```python
from build123d import *

# Parameters (mm, degrees)
SKETCH_1_R      = 1.3
EXTRUDE_1_DEPTH = 1.6
EXTRUDE_2_DEPTH = 6
SKETCH_3_W      = 6
SKETCH_3_H      = 6
EXTRUDE_3_DEPTH = 0.6
SKETCH_4_W      = 1.6
SKETCH_4_H      = 1.6
EXTRUDE_4_DEPTH = 0.6
SKETCH_5_W      = 32.8
SKETCH_5_H      = 9.5
EXTRUDE_5_DEPTH = 8


with BuildPart() as part:
    # 草图1 → 凸台-拉伸1 (new body)
    with BuildSketch(Plane(origin=(0, 0, 0), x_dir=(1, 0, 0), z_dir=(0, 1, 0))):
        with BuildLine():
            Line((-12, -17.5), (12, -17.5))
            ThreePointArc((12, -17.5), (12.707106781, -17.207106781), (13, -16.5))
            Line((13, -16.5), (13, 16.5))
            ThreePointArc((13, 16.5), (12.707106781, 17.207106781), (12, 17.5))
            Line((12, 17.5), (-12, 17.5))
            ThreePointArc((-12, 17.5), (-12.707106781, 17.207106781), (-13, 16.5))
            Line((-13, 16.5), (-13, -16.5))
            ThreePointArc((-13, -16.5), (-12.707106781, -17.207106781), (-12, -17.5))
        make_face()
        with Locations((-11, -15.5)):
            Circle(SKETCH_1_R, mode=Mode.SUBTRACT)
        with Locations((11, 15.5)):
            Circle(SKETCH_1_R, mode=Mode.SUBTRACT)
    extrude(amount=EXTRUDE_1_DEPTH)

    # 草图2 → 凸台-拉伸2 (add)
    with BuildSketch(Plane.ZY.offset(13)):
        with BuildLine():
            Line((-3.4, 3.2), (3.4, 3.2))
            ThreePointArc((3.4, 3.2), (5, 1.6), (3.4, 0))
            Line((3.4, 0), (-3.4, 0))
            ThreePointArc((-3.4, 0), (-5, 1.6), (-3.4, 3.2))
        make_face()
    extrude(amount=-EXTRUDE_2_DEPTH)

    # 草图3 → 凸台-拉伸3 (add)
    with BuildSketch(Plane(origin=(0, 1.6, 0), x_dir=(1, 0, 0), z_dir=(0, 1, 0))):
        with Locations((0.65, 0)):
            Rectangle(SKETCH_3_W, SKETCH_3_H)
    extrude(amount=EXTRUDE_3_DEPTH)

    # 草图4 → 凸台-拉伸4 (add)
    with BuildSketch(Plane(origin=(0, 1.6, 0), x_dir=(1, 0, 0), z_dir=(0, 1, 0))):
        with Locations((8.15, 0)):
            Rectangle(SKETCH_4_W, SKETCH_4_H)
    extrude(amount=EXTRUDE_4_DEPTH)

    # 草图5 → 凸台-拉伸5 (add)
    with BuildSketch(Plane(origin=(13, 0, 0), x_dir=(0, 0, -1), z_dir=(1, 0, 0))):
        with Locations((0, 0.8)):
            Rectangle(SKETCH_5_W, SKETCH_5_H)
    extrude(amount=EXTRUDE_5_DEPTH)


solid = part.part
```
CAD build for the part. Positions are in the model's coordinates, mm. A direction names the side the tool comes from. Round coordinates to 2 decimals unless told otherwise and drop trailing zeros. Write each loop counter-clockwise with the first axis right and the second up, starting at its lowest first coordinate (ties: lowest second). Pieces come first, ordered by that corner, then holes. Notation, with made-up numbers: (-32.75, -37.75) - (18.25, -37.75) arc R11 ccw to (18.25, -20.75) - close; hole circle Ø6 at (29, 64). An arc over 180 degrees is marked (long way). Write item = value, one per line. Start each with the question number.
Q1. Drop flat-ended pins along their axis: pin 1 (0.8 mm diameter, centred on x = 8, z = 0.5, fed in from +Y); pin 2 (4 mm diameter, centred on x = 16, y = 1.5, fed in from +Z); pin 3 (0.5 mm diameter, centred on x = -1, y = 2, fed in from +Z). Give the stop position or say it passes through.
Q2. Band-saw the part on B-B (x = -11). Give the cut face in (y, z), then the cut area to 3 significant figures.
Q3. Band-saw the part on D-D (x = 11). Give the cut face in (y, z).
Q4. Band-saw the part on A-A (z = -15.5). Give the cut face in (x, y).
Q5. Band-saw the part on C-C (z = -6). Give the cut face in (x, y), then the cut area to 3 significant figures.
Q6. Probe L1, parallel to X at y = 1.1, z = -15.5; L2, parallel to Z at x = 11, y = 1; L3, parallel to Z at x = -11, y = 1.05. List the from-to ranges inside material, lowest first. Write a range as from..to.
Q7. Mould opens along X. For faces 4 (the flat face through (13, 4, 0)), 5 (the flat face through (13, -2, 0)), 6 (the cylindrical face through (-10.04, 2.74, 4.52)), 7 (the flat face through (21, 1, 0)) say: pulls with the +X half, pulls with the -X half, needs draft (parallel to the pull), parting line crosses it, or undercut.
Q8. Which spindle directions (+Z, -Z, +X, -X, +Y, -Y) get a long thin tool onto all of the face, cutting with end or side? Do faces 1 (the cylindrical face through (-10.04, 2.72, -4.54)), 2 (the flat face through (-7, 2, 0)), 3 (the flat face through (17, -3.95, 0)). Say none if no direction does.
Answers below:
q1.pin_1 = 2.2
q1.pin_2 = 16.4
q1.pin_3 = 3
q2.outline = (0, -17.5) - (1.6, -17.5) - (1.6, -5) arc R1.6 ccw to (3.2, -3.4) - (3.2, 3.4) arc R1.6 ccw to (1.6, 5) - (1.6, 14.2) - (0, 14.2) - close; (0, 16.8) - (1.6, 16.8) - (1.6, 17.5) - (0, 17.5) - close
q2.area = 66.7 mm2
q3.outline = (0, -17.5) - (1.6, -17.5) - (1.6, -16.8) - (0, -16.8) - close; (0, -14.2) - (1.6, -14.2) - (1.6, 17.5) - (0, 17.5) - close
q4.outline = (-13, 0) - (9.7, 0) - (9.7, 1.6) - (-13, 1.6) - close; (12.3, 0) - (13, 0) - (13, -3.95) - (21, -3.95) - (21, 5.55) - (13, 5.55) - (13, 1.6) - (12.3, 1.6) - close
q5.outline = (-13, 0) - (13, 0) - (13, -3.95) - (21, -3.95) - (21, 5.55) - (13, 5.55) - (13, 1.6) - (-13, 1.6) - close
q5.area = 118 mm2
q6.L1 = -13..9.7, 12.3..21
q6.L2 = -17.5..-16.8, -14.2..17.5
q6.L3 = -17.5..14.2, 16.8..17.5
q7.face_4 = undercut
q7.face_5 = pulls with the -X half
q7.face_6 = needs draft
q7.face_7 = pulls with the +X half
q8.face_1 = -Z, -X, +Y
q8.face_2 = +Z, -Z, +Y
q8.face_3 = +Z, -Z, +X, -X, -Y
